Verification items for the finished model (mm, model axes). A direction names the side the tool comes from. Round coordinates to 2 decimals unless told otherwise and drop trailing zeros. Write each loop counter-clockwise with the first axis right and the second up, starting at its lowest first coordinate (ties: lowest second). Pieces come first, ordered by that corner, then holes. Notation, with made-up numbers: (-19.5, -3.5) - (-4.5, -3.5) arc R22 cw to (-4.5, 10.5) - close; hole circle Ø10 at (-0.75, 26). An arc over 180 degrees is marked (long way). Answer as a JSON object with one key per item and string values. Group by question number.
1) Section check C-C (y = 1.75). Enter the section's corners in (x, z), then the cut area to 3 significant figures.
2) Section check B-B (z = 0). Enter the section's corners in (x, y), then the cut area to 3 significant figures.
3) Thickness scan on line 1 (Z direction, x = 0, y = 0.95); line 2 (Y direction, x = -2.5, z = 1.5); line 3 (Y direction, x = -4, z = 0.5). Record the ranges inside material, lowest first.
4) Section check A-A (x = 0). Enter the section's corners in (y, z).
5) Go/stop test with a flat-tipped pin: pin 1 Ø1.5 at (x, z) = (2.5, -3) entering from +Y. Record where the tip stops, or that it passes through.
6) Mould release check, pull along X, two halves, no side actions. Record for faces 4 (the cylindrical face through (-1.5, 7.95, -0.07)), 5 (the flat face through (0, 2.46, 0)), 6 (the flat face through (1.4, 0, 1.4)), 7 (the cylindrical face through (1.617, 1.213, -0.67)): +X half, -X half, draft (parallel to the pull), parting line (faces both ways), or undercut.
7) Set-up check for faces 1 (the cylindrical face through (-2.579, 1.213, 1.978)), 2 (the flat face through (0, 8.46, 0)), 3 (the flat face through (2, 7.46, 0)): record each of +Z, -Z, +X, -X, +Y, -Y from which the full face is reachable in a straight line by a thin tool's end or side.
8) Section check D-D (y = 5.5). Enter the section's corners in (x, z).
```python
from build123d import *

# Parameters (mm, degrees)
SKETCH1_R           = 3.25
BOSS_EXTRUDE1_DEPTH = 2.46
SKETCH2_R           = 1.75
CUT_EXTRUDE1_DEPTH  = 2.5
SKETCH6_R           = 4.8
BOSS_EXTRUDE2_DEPTH = 5
FILLET2_R           = 0.75
SKETCH7_R           = 1.5
BOSS_EXTRUDE3_DEPTH = 1


with BuildPart() as part:
    # Sketch1 → Boss-Extrude1 (new body)
    with BuildSketch(Plane(origin=(0, 0, 0), x_dir=(1, 0, 0), z_dir=(0, 1, 0))):
        Circle(SKETCH1_R)
    extrude(amount=BOSS_EXTRUDE1_DEPTH)

    # Sketch2 → Cut-Extrude1 (cut)
    with BuildSketch(Plane.XZ):
        Circle(SKETCH2_R)
    extrude(amount=-CUT_EXTRUDE1_DEPTH, mode=Mode.SUBTRACT)

    # Sketch6 → Boss-Extrude2 (add)
    with BuildSketch(Plane(origin=(0, 2.46, 0), x_dir=(1, 0, 0), z_dir=(0, 1, 0))):
        Circle(SKETCH6_R)
    extrude(amount=BOSS_EXTRUDE2_DEPTH)

    # Fillet2
    fillet2_edges = [part.edges().sort_by_distance(p)[0] for p in [
        (-4.8, 7.46, 0),
    ]]
    fillet(fillet2_edges, radius=FILLET2_R)

    # Sketch7 → Boss-Extrude3 (add)
    with BuildSketch(Plane(origin=(0, 7.46, 0), x_dir=(1, 0, 0), z_dir=(0, 1, 0))):
        Circle(SKETCH7_R)
    extrude(amount=BOSS_EXTRUDE3_DEPTH)


solid = part.part
```
Returned:
{
 "1": {"outline": "circle Ø6.5 at (0, 0); hole circle Ø3.5 at (0, 0)", "area": "23.6 mm2"},
 "2": {"outline": "(-4.8, 2.46) - (-3.25, 2.46) - (-3.25, 0) - (-1.75, 0) - (-1.75, 2.46) - (1.75, 2.46) - (1.75, 0) - (3.25, 0) - (3.25, 2.46) - (4.8, 2.46) - (4.8, 6.71) arc R0.75 ccw to (4.05, 7.46) - (1.5, 7.46) - (1.5, 8.46) - (-1.5, 8.46) - (-1.5, 7.46) - (-4.05, 7.46) arc R0.75 ccw to (-4.8, 6.71) - close", "area": "58.1 mm2"},
 "3": {"line 1": "-3.25 to -1.75, 1.75 to 3.25", "line 2": "0 to 7.46", "line 3": "2.46 to 7.46"},
 "4": {"outline": "(0, -3.25) - (2.46, -3.25) - (2.46, -4.8) - (6.71, -4.8) arc R0.75 ccw to (7.46, -4.05) - (7.46, -1.5) - (8.46, -1.5) - (8.46, 1.5) - (7.46, 1.5) - (7.46, 4.05) arc R0.75 ccw to (6.71, 4.8) - (2.46, 4.8) - (2.46, 3.25) - (0, 3.25) - (0, 1.75) - (2.46, 1.75) - (2.46, -1.75) - (0, -1.75) - close"},
 "5": {"pin 1": "y = 7.46"},
 "6": {"face 4": "parting line", "face 5": "undercut", "face 6": "draft", "face 7": "undercut"},
 "7": {"face 1": "-Y", "face 2": "+Z, -Z, +X, -X, +Y", "face 3": "+Y"},
 "8": {"outline": "circle Ø9.6 at (0, 0)"}
}
